Geometry: final body of the model. Coordinates: model frame, mm. A direction names the side the tool comes from. Round coordinates to 2 decimals unless told otherwise and drop trailing zeros. Order: outer loops, then holes, each group sorted by start corner. A loop starts at its lowest first (then second) coordinate and runs counter-clockwise, first axis right, second up. Notation, with made-up numbers: (58, 84.25) -> (110, 84.25) arc R13 cw to (110, 101.25) -> close; hole circle Ø5 at (59, 74). An arc over 180 degrees is marked (long way). Put each result on its own line as item: value.
```python
from build123d import *

# Parameters (mm, degrees)
SKETCH1_W           = 200
SKETCH1_H           = 45
BOSS_EXTRUDE1_DEPTH = 17.45
FILLET1_R           = 18
FILLET2_R           = 23
SKETCH2_W           = 40
SKETCH2_H           = 45
CUT_EXTRUDE1_DEPTH  = 7.5
SKETCH3_R           = 6
CUT_EXTRUDE2_DEPTH  = 120.515065654
SKETCH4_R           = 6
CUT_EXTRUDE3_DEPTH  = 124.027462877
SCALE1_SCALE        = 0.31


with BuildPart() as part:
    # Sketch1 → Boss-Extrude1 (new, symmetric)
    with BuildSketch(Plane(origin=(0, 0, 0), x_dir=(1, 0, 0), z_dir=(0, 1, 0))):
        with Locations((13.173125929, -4.459910913)):
            Rectangle(SKETCH1_W, SKETCH1_H)
    extrude(amount=BOSS_EXTRUDE1_DEPTH, both=True)

    # Fillet1
    # the kernel refuses this fillet: 18 mm, written as the material it takes off along each edge
    with BuildSketch(Plane(origin=(113.173125929, -17.45, -63.040089087), x_dir=(0, 1, 0), z_dir=(0, 0, 1)), Plane(origin=(113.173125929, 17.45, -63.040089087), x_dir=(-1, 0, 0), z_dir=(0, 0, 1))) as fillet1_piece_1:
        with BuildLine():
            CenterArc((FILLET1_R, FILLET1_R), FILLET1_R, 180, 90)
            Line((0, FILLET1_R), (0, 0))
            Line((0, 0), (FILLET1_R, 0))
        make_face()
    extrude(amount=135, mode=Mode.SUBTRACT)

    # Fillet2
    # the kernel refuses this fillet: 23 mm, written as the material it takes off along each edge
    with BuildSketch(Plane(origin=(-86.826874071, -74.95, -18.040089087), x_dir=(1, 0, 0), z_dir=(0, 1, 0)), Plane(origin=(-86.826874071, -74.95, 26.959910913), x_dir=(0, 0, -1), z_dir=(0, 1, 0))) as fillet2_piece_1:
        with BuildLine():
            CenterArc((FILLET2_R, -FILLET2_R), FILLET2_R, 90, 90)
            Line((0, -FILLET2_R), (0, 0))
            Line((0, 0), (FILLET2_R, 0))
        make_face()
    extrude(amount=149.9, mode=Mode.SUBTRACT)

    # Sketch2 → Cut-Extrude1 (cut)
    with BuildSketch(Plane(origin=(0, 17.45, 0), x_dir=(1, 0, 0), z_dir=(0, 1, 0))):
        with Locations((-70.821438646, -4.459910913)):
            Rectangle(SKETCH2_W, SKETCH2_H)
    cut_extrude1 = extrude(amount=-CUT_EXTRUDE1_DEPTH, mode=Mode.SUBTRACT)

    # Mirror1: Cut-Extrude1 across plane
    add(cut_extrude1.mirror(Plane.ZX), mode=Mode.SUBTRACT)

    # Sketch3 → Cut-Extrude2 (cut, through all)
    with BuildSketch(Plane(origin=(0, 9.95, 0), x_dir=(1, 0, 0), z_dir=(0, 1, 0))):
        with Locations(Location((-72.821438646, -3.356394194, 0), (0, 0, 270))):
            Circle(SKETCH3_R)
    extrude(amount=-CUT_EXTRUDE2_DEPTH, mode=Mode.SUBTRACT)

    # Sketch4 → Cut-Extrude3 (cut, through all)
    with BuildSketch(Plane.XY.offset(26.959910913)):
        with Locations((98.164721189, 0)):
            Circle(SKETCH4_R)
    extrude(amount=-CUT_EXTRUDE3_DEPTH, mode=Mode.SUBTRACT)


with BuildPart() as part_1:
    # Scale1: scaled about (0, 0, 0)
    add(part.part.scale(SCALE1_SCALE))


solid = part_1.part
```
1. Cut plane B-B on z = 2.25. Return loops of the section in (x, y).
Ans:
outline: (-26.84, -3.08) -> (-23.99, -3.08) -> (-23.99, 3.08) -> (-26.84, 3.08) -> close; (-21.16, -3.08) -> (-15.75, -3.08) -> (-15.75, -5.41) -> (29.5, -5.41) arc R5.58 ccw to (35.08, 0) arc R5.58 ccw to (29.5, 5.41) -> (-15.75, 5.41) -> (-15.75, 3.08) -> (-21.16, 3.08) -> close; hole circle Ø3.72 at (30.43, 0)
2. Material intervals for probe 1 along Y at (x, z) = (-20, -2.75); probe 2 along X at (y, z) = (0.5, 5.5); probe 3 along X at (y, z) = (-0.25, 3.5), sorted ascending.
Ans:
probe 1: -3.08 to 3.08
probe 2: -25.49 to 28.64, 32.22 to 35.04
probe 3: -26.54 to 28.59, 32.27 to 35.07
3. Cut plane A-A on y = -1. Return loops of the section in (x, z).
Ans:
outline: (-26.91, 1.38) arc R7.13 ccw to (-19.79, -5.59) -> (28.86, -5.59) -> (28.86, 8.36) -> (-19.79, 8.36) arc R7.13 ccw to start; (32, -5.59) -> (34.96, -5.59) -> (34.96, 8.36) -> (32, 8.36) -> close; hole circle Ø3.72 at (-22.57, 1.04)
4. Cut plane C-C on z = -4.5. Return loops of the section in (x, y), and give its area (3 significant figures).
Ans:
outline: (-23.58, -3.08) -> (-15.75, -3.08) -> (-15.75, -5.41) -> (29.5, -5.41) arc R5.58 ccw to (35.08, 0) arc R5.58 ccw to (29.5, 5.41) -> (-15.75, 5.41) -> (-15.75, 3.08) -> (-23.58, 3.08) -> close; hole circle Ø3.72 at (30.43, 0)
area: 574 mm²
5. Draft query along Y for faces 4 (the face through (32, 1, 1)), 5 (the face through (7, 0, -5.592)), 6 (the face through (7, -5.409, 1)). Return one class per face: +Y half, -Y half, draft (parallel to the pull), parting line (faces both ways), or undercut.
Ans:
face 4: undercut
face 5: draft
face 6: -Y half
6. Cut plane D-D on x = -17.5. Return loops of the section in (y, z), and give its area (3 significant figures).
Ans:
outline: (-3.08, -5.59) -> (3.08, -5.59) -> (3.08, 8.36) -> (-3.08, 8.36) -> close
area: 86.1 mm²
7. Contact query for flat-ended pins moving along their axis: P1, Ø5, axis at x = -22.57, z = 1.04, coming from the +Y side; P2, Ø1.9, axis at y = 4, z = 1, coming from the -X side; P3, Ø1.9, axis at y = -3.5, z = -1, coming from the -X side. Output: stop coordinate, or through.
Ans:
P1: y = 3.08
P2: x = -26.91
P3: x = -26.71
8. Set-up query: faces 1 (the face through (-20, 3.085, 1)), 2 (the face through (-15.755, -4, 1)), 3 (the face through (-24.39, 0.04, 0.64)). Return all of +Z, -Z, +X, -X, +Y, -Y with unobstructed straight access to the full face (end or side cutting, diameter ignored); none if empty.
Ans:
face 1: +Z, -Z, -X, +Y
face 2: +Z, -Z, -X, -Y
face 3: +Y, -Y
